The model under review builds one solid part; all positions refer to its coordinate system, in mm. Round coordinates to 2 decimals unless told otherwise and drop trailing zeros. Order: outer loops, then holes, each group sorted by start corner. A loop starts at its lowest first (then second) coordinate and runs counter-clockwise, first axis right, second up. Notation, with made-up numbers: M 59,-35 L 81,-35 A11 ccw 81,-27 Z; hole C -33,-23 d11. An arc over 180 degrees is marked long. Answer as a JSON object with one key per item and string values. Group by question number.
1. Add section C-C on z = -7. State the section outline as (x, y) points, and give its area (3 significant figures).
2. Add section B-B on x = 23.25. State the section outline as (y, z) points.
3. Clearance check with flat-ended pins moving along their axes: P1, Ø3, axis at x = 10, y = 5.5, coming from the -Z side; P2, Ø1, axis at x = 9, y = 20.5, coming from the -Z side; P3, Ø3, axis at y = 14.5, z = -10, coming from the +X side. State where each tip first meets the part, or that it passes through.
4. Add section A-A on y = 2.5. State the section outline as (x, z) points.
5. To check wall thickness, follow probe 1 along Z at (x, y) = (20.5, 23.75); probe 2 along Z at (x, y) = (10.5, 23); probe 3 along Z at (x, y) = (14.75, 23.75). State the ranges of each line that lie inside material, in increasing order. Write a range as [from, to].
6. Mouldability with a two-part tool opening along Z and no side actions: class faces 1 (the face through (12, 25, 5)), 2 (the face through (4, 18.2, 0)), 3 (the face through (12, 13, 10)) as released by +Z, released by -Z, zero draft, split by the parting line, or undercut.
7. Add section D-D on x = 9. State the section outline as (y, z) points, and give its area (3 significant figures).
```python
from build123d import *

# Parameters (mm, degrees)
SKETCH1_W           = 25
SKETCH1_H           = 25
BOSS_EXTRUDE1_DEPTH = 10


with BuildPart() as part:
    # Sketch1 → Boss-Extrude1 (new body)
    with BuildSketch(Plane.XY):
        with Locations((12.5, 12.5)):
            Rectangle(SKETCH1_W, SKETCH1_H)
    extrude(amount=BOSS_EXTRUDE1_DEPTH)

    # Sketch3 → Revolve1 (revolve)
    with BuildSketch(Plane(origin=(0, 12.5, 0), x_dir=(-1, 0, 0), z_dir=(0, -1, 0))):
        with BuildLine():
            Line((-12.5, 20), (-12.5, -5))
            ThreePointArc((-12.5, -5), (0, 7.5), (-12.5, 20))
        make_face()
    revolve(axis=Axis((12.5, 12.5, 0), (0, 0, 1)))


solid = part.part
```
Recorded:
{
 "1": {"outline": "C 12.5,12.5 d24.98", "area": "490 mm²"},
 "2": {"outline": "M 0,0 L 25,0 L 25,10 L 0,10 Z; C 12.5,-7.5 d12.76"},
 "3": {"P1": "stops at z = -18.5", "P2": "stops at z = -16.91", "P3": "stops at x = 24.88"},
 "4": {"outline": "M 0,0 L 25,0 L 25,10 L 0,10 Z; C 12.5,-7.5 d15"},
 "5": {"probe 1": "z = [0, 10]", "probe 2": "z = [-13.98, -1.02], [0, 10]", "probe 3": "z = [-12.46, -2.54], [0, 10]"},
 "6": {"face 1": "zero draft", "face 2": "undercut", "face 3": "released by +Z"},
 "7": {"outline": "M 0,0 L 3.13,0 A12 ccw long 21.87,0 L 25,0 L 25,10 L 0,10 Z", "area": "644 mm²"}
}
